Source: CAD feature listing. Evaluate the final solid. Frame: model axes, mm. Face numbers are marked on the shaded views. Give positions to 0.01 mm unless a question says otherwise; leave off trailing zeros. Order: outer loops, then holes, each group sorted by start corner. A loop starts at its lowest first (then second) coordinate and runs counter-clockwise, first axis right, second up.
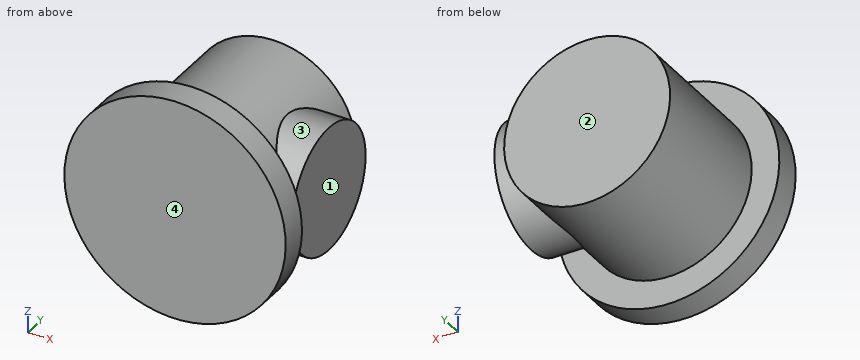
from build123d import *

# Parameters (mm, degrees)
SKETCH1_R           = 50.8
SKETCH1_R_2         = 38.1
BOSS_EXTRUDE1_DEPTH = 12.7
BOSS_EXTRUDE2_START = 12.7
SKETCH1_3_R         = 38.1
BOSS_EXTRUDE2_DEPTH = 63.5
SKETCH2_R           = 28.575
BOSS_EXTRUDE3_DEPTH = 44.45


with BuildPart() as part:
    # Sketch1 → Boss-Extrude1 (new body)
    with BuildSketch(Plane(origin=(0, 0, 0), x_dir=(1, 0, 0), z_dir=(0, 1, 0))):
        with Locations(Location((0, 0, 0), (0, 0, 270))):
            Circle(SKETCH1_R)
        Circle(SKETCH1_R_2, mode=Mode.SUBTRACT)
        Circle(SKETCH1_R_2)
    extrude(amount=BOSS_EXTRUDE1_DEPTH)

    # Sketch1<3> → Boss-Extrude2 (add)
    with BuildSketch(Plane(origin=(0, 0, 0), x_dir=(1, 0, 0), z_dir=(0, 1, 0)).offset(BOSS_EXTRUDE2_START)):
        with Locations(Location((0, 0, 0), (0, 0, 270))):
            Circle(SKETCH1_3_R)
    extrude(amount=BOSS_EXTRUDE2_DEPTH)

    # Sketch2 → Boss-Extrude3 (add)
    with BuildSketch(Plane(origin=(0, 0, 0), x_dir=(0, 0, -1), z_dir=(1, 0, 0))):
        with Locations(Location((0, 44.45, 0), (0, 0, 180))):
            Circle(SKETCH2_R)
    extrude(amount=BOSS_EXTRUDE3_DEPTH)


solid = part.part
(1) Pin query (flat end, axial travel): pin 1 Ø4 at (y, z) = (19, -6.5) entering from -X; pin 2 Ø12 at (x, z) = (-8.5, -38) entering from -Y; pin 3 Ø5 at (y, z) = (64.5, 21.5) entering from +X; pin 4 Ø8 at (y, z) = (29.5, -12) entering from -X. Return the tip coordinate at first contact, or that it passes through.
(2) Section B-B, the plane x = 0. Return loops of the section in (y, z), plus the area to 3 significant figures.
(3) Section A-A, the plane z = 0. Return loops of the section in (x, y) (3 decimals), plus the area to 3 significant figures.
(4) Draft query along Y for the marked faces 1, 2, 3 and 4. Return one class per face: +Y half, -Y half, draft (parallel to the pull), parting line (faces both ways), or undercut.
(5) Section D-D, the plane x = -23.5. Return loops of the section in (y, z).
(6) Section C-C, the plane y = 44.45. Return loops of the section in (x, z) (3 decimals).
(7) Line query: line 1 along Y through (x, z) = (-36.5, 25.5); line 2 along Z through (x, y) = (31, 45); line 3 along X through (y, z) = (57, 33.5). Output: solid intervals per line, ascending.
Checks:
1. pin 1: stops at x = -37.83
1. pin 2: stops at y = 0
1. pin 3: stops at x = 44.45
1. pin 4: stops at x = -37.25
2. outline: (0, -50.8) - (12.7, -50.8) - (12.7, -38.1) - (76.2, -38.1) - (76.2, 38.1) - (12.7, 38.1) - (12.7, 50.8) - (0, 50.8) - close
2. area: 6,130 mm2
3. outline: (-50.8, 0) - (50.8, 0) - (50.8, 12.7) - (38.1, 12.7) - (38.1, 15.875) - (44.45, 15.875) - (44.45, 73.025) - (38.1, 73.025) - (38.1, 76.2) - (-38.1, 76.2) - (-38.1, 12.7) - (-50.8, 12.7) - close
3. area: 6,490 mm2
4. face 1: draft
4. face 2: +Y half
4. face 3: undercut
4. face 4: -Y half
5. outline: (0, -45.04) - (12.7, -45.04) - (12.7, -29.99) - (76.2, -29.99) - (76.2, 29.99) - (12.7, 29.99) - (12.7, 45.04) - (0, 45.04) - close
6. outline: (25.201, -28.575) - (44.45, -28.575) - (44.45, 28.575) - (25.201, 28.575) arc R38.1 ccw (long way) to start
7. line 1: y = 0 to 12.7
7. line 2: z = -28.57 to 28.57
7. line 3: x = -18.15 to 18.15
